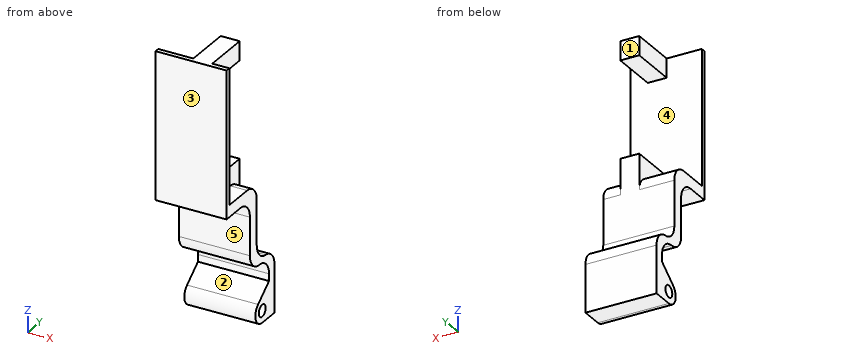
Autodesk Inventor part; units mm, degrees
ref_plane "作業平面1" through (7.8, 0, 0) normal (1, 0, 0) x (0, 0, -1)
ref_plane "YZ Plane" through (0, 0, 0) normal (1, 0, 0) x (0, 1, 0)
ref_plane "XZ Plane" through (0, 0, 0) normal (0, 1, 0) x (-1, 0, 0)
sketch "スケッチ1" plane through (0, 0, 0) normal (0, 1, 0) x (-1, 0, 0)
  line L0 (15, 0) -> (-15, 0)
  line L1 (-15, 0) -> (-15, -56.8)
  line L2 (-15, -56.8) -> (15, -56.8)
  line L3 (15, -56.8) -> (15, 0)
  point P0 (0, 0)
  point P1 (0, 0)
  dimension "d0" = 30
  dimension "d9" = 56.8
extrude "押し出し1" add sketch "スケッチ1" along normal blind 2
ref_plane "作業平面1" through (7.8, 0, 0) normal (1, 0, 0) x (0, 0, -1)
sketch "スケッチ2" plane through (7.8, 0, 0) normal (1, 0, 0) x (0, 0, -1)
  line L0 (0, 2) -> (56.8, 2)
  line L1 (56.8, 2) -> (56.8, 22.1)
  line L2 (56.8, 22.1) -> (0, 22.1)
  line L3 (0, 22.1) -> (0, 2)
  line L4 (8, 2) -> (48.8, 2)
  line L5 (48.8, 2) -> (48.8, 22.1)
  line L6 (48.8, 22.1) -> (8, 22.1)
  line L7 (8, 22.1) -> (8, 2)
  line L8 (0, 2) -> (56.8, 2)
  line L9 (0, 0) -> (0, 2)
  point P0 (28.4, 22.1)
  dimension "d4" = 56.8
  dimension "d5" = 40.8
  dimension "d6" = 20.1
extrude "押し出し2" add sketch "スケッチ2" against normal blind 8 contours L3 L2 L7 L0 | L5 L2 L1 L0
sketch "スケッチ3" plane through (15, 0, -56.8) normal (0, 0, -1) x (-1, 0, 0)
  line L0 (30, 0) -> (0, 0)
  line L1 (0, 0) -> (30, 0)
  line L2 (30, 0) -> (30, 22.1)
  line L3 (30, 22.1) -> (0, 22.1)
  line L4 (0, 22.1) -> (0, 0)
  line L5 (7.2, 22.1) -> (15.2, 22.1)
  line L6 (30, 0) -> (30, 2)
  point P0 (15, 0)
extrude "押し出し3" add sketch "スケッチ3" along normal blind 5
sketch "スケッチ4" plane through (15, 0, -61.8) normal (0, 0, -1) x (-1, 0, 0)
  line L0 (7.2, 22.1) -> (0, 22.1)
  line L1 (30, 2) -> (30, 22.1)
  line L2 (0, 22.1) -> (30, 22.1)
  line L3 (30, 22.1) -> (30, 17.1)
  line L4 (30, 17.1) -> (0, 17.1)
  line L5 (0, 17.1) -> (0, 22.1)
  point P0 (15, 0)
  point P1 (7.2, 22.1)
  dimension "d12" = 5
extrude "押し出し4" add sketch "スケッチ4" along normal blind 28
sketch "スケッチ5" plane through (15, 0, -89.8) normal (0, 0, -1) x (-1, 0, 0)
  line L0 (0, 17.1) -> (30, 17.1)
  line L1 (0, 17.1) -> (30, 17.1)
  line L2 (30, 17.1) -> (30, 35.1)
  line L3 (30, 35.1) -> (0, 35.1)
  line L4 (0, 35.1) -> (0, 17.1)
  line L5 (30, 17.1) -> (30, 22.1)
  line L6 (30, 22.1) -> (0, 22.1)
  point P0 (15, 0)
  dimension "d21" = 13
extrude "押し出し5" add sketch "スケッチ5" along normal blind 2
sketch "スケッチ6" plane through (15, 0, -91.8) normal (0, 0, -1) x (-1, 0, 0)
  line L0 (30, 22.1) -> (30, 35.1)
  line L1 (0, 35.1) -> (30, 35.1)
  line L2 (30, 35.1) -> (30, 31.1)
  line L3 (30, 31.1) -> (0, 31.1)
  line L4 (0, 31.1) -> (0, 35.1)
  line L5 (0, 35.1) -> (0, 17.1)
  line L6 (30, 35.1) -> (0, 35.1)
  point P0 (15, 0)
  point P1 (30, 35.1)
  dimension "d18" = 4
extrude "押し出し6" add sketch "スケッチ6" along normal blind 25
fillet "フィレット1" radius 7 7 edges at (0, 17.1, -61.8) (0, 17.1, -91.8) (0, 31.1, -91.8) (0, 22.1, -89.8) (0, 35.1, -89.8) (11.4, 22.1, -56.8) (-7.6, 22.1, -56.8)
sketch "スケッチ7" plane through (15, 0, 0) normal (1, 0, 0) x (0, 0, -1)
  circle A0 centre (111.8, 26.1) radius 5
  circle A1 centre (111.8, 26.1) radius 2.5
  line L0 (98.8, 31.1) -> (116.8, 31.1)
  line L1 (116.8, 35.1) -> (116.8, 31.1)
  line L2 (116.8, 31.1) -> (116.8, 26.1)
  line L3 (101.8, 31.1) -> (107.8, 23.1)
  point P0 (0, 0)
  dimension "d23" = 10
  dimension "d24" = 5
  dimension "d25" = 10
extrude "押し出し7" add sketch "スケッチ7" against normal up to surface (30 mm away)
properties part number "arm_0"
Input: part model. Units: mm. Frame: model coordinates. Face numbers are marked on the shaded views. A direction names the side the tool comes from. Round coordinates to 2 decimals unless told otherwise and drop trailing zeros. Loops run counter-clockwise (first coordinate to the right, second up) from the corner with the lowest first, then second, coordinate; pieces in that order, holes last. Notation, with made-up numbers: M -35,10.25 L 17,10.25 A17 cw 17,31.25 Z; hole C -22,-8.75 d3. An arc over 180 degrees is marked long. Answer in a Markdown table with one row per item. Add a question column.
1. Ray query, probe 1 along Y at (x, z) = (2, -111.8); probe 2 along Z at (x, y) = (4, 26) (3 decimals); probe 3 along Z at (x, y) = (13.5, 24) (3 decimals). Return the intervals inside material, ascending.
2. Section A-A (y = 7). Output: boundary loops of the cut face in (x, z), and give its area (3 significant figures).
3. Section C-C (y = 19). Output: boundary loops of the cut face in (x, z).
4. Contact query for flat-ended pins moving along their axis: pin 1 (3.5 mm diameter, centred on x = 1.5, z = -100, fed in from -Y); pin 2 (1.5 mm diameter, centred on x = -10.5, z = -77.5, fed in from +Y); pin 3 (5 mm diameter, centred on x = 5.5, z = -80, fed in from -Y); pin 4 (4 mm diameter, centred on y = 26.1, z = -111.8, fed in from +X). Output: stop coordinate, or through.
5. Mould query, pull axis Z, two halves, no side actions, for the marked faces 4 and 5. Classes: released by +Z, released by -Z, zero draft, split by the parting line, or undercut.
6. Section D-D (z = -44). Output: boundary loops of the cut face in (x, y).
7. Set-up query: the marked faces 1, 2 and 3. Return all of +Z, -Z, +X, -X, +Y, -Y with unobstructed straight access to the full face (end or side cutting, diameter ignored); none if empty.
8. Section B-B (z = -111.8). Output: boundary loops of the cut face in (x, y).
Values follow:
| question | item | result |
|---|---|---|
| 1 | probe 1 | 21.1 to 23.6, 28.6 to 35.1 |
| 1 | probe 2 | -116.799 to -114.298, -109.302 to -105.625, -92.063 to -89.076 |
| 1 | probe 3 | -116.338 to -113.156, -110.444 to -107.125, -91.799 to -87.595 |
| 2 | outline | M -15,-61.8 L 15,-61.8 L 15,-56.8 L 7.8,-56.8 L 7.8,-48.8 L -0.2,-48.8 L -0.2,-56.8 L -15,-56.8 Z; M -0.2,-8 L 7.8,-8 L 7.8,0 L -0.2,0 Z |
| 2 | area | 278 mm^2 |
| 3 | outline | M -15,-89.59 L 15,-89.59 L 15,-57.99 L 7.8,-57.99 L 7.8,-48.8 L -0.2,-48.8 L -0.2,-57.99 L -15,-57.99 Z; M -0.2,-8 L 7.8,-8 L 7.8,0 L -0.2,0 Z |
| 4 | pin 1 | y = 31.08 |
| 4 | pin 2 | y = 22.1 |
| 4 | pin 3 | y = 17.1 |
| 4 | pin 4 | through |
| 5 | face 4 | undercut |
| 5 | face 5 | zero draft |
| 6 | outline | M -15,0 L 15,0 L 15,2 L -15,2 Z |
| 7 | face 1 | +Z, +X, -X, +Y |
| 7 | face 2 | +X, -X, -Y |
| 7 | face 3 | +Z, -Z, +X, -X, -Y |
| 8 | outline | M -15,21.1 L 15,21.1 L 15,23.6 L -15,23.6 Z; M -15,28.6 L 15,28.6 L 15,35.1 L -15,35.1 Z |
